Input: part model. Units: mm. Frame: model coordinates. Round coordinates to 2 decimals unless told otherwise and drop trailing zeros. Order: outer loops, then holes, each group sorted by start corner. A loop starts at its lowest first (then second) coordinate and runs counter-clockwise, first axis right, second up. Notation, with made-up numbers: (6.25, 47.25) -> (36.25, 47.25) arc R35 cw to (36.25, 84.25) -> close; hole circle Ø2 at (70.25, 43.5). An arc over 180 degrees is marked (long way). Use a Markdown table: item, result.
from build123d import *

# Parameters (mm, degrees)
ESQUISSE1_W                = 80
ESQUISSE1_H                = 30
BOSS_EXTRU_1_DEPTH         = 3
ESQUISSE2_W                = 10
ESQUISSE2_H                = 3
ENL_V_MAT_EXTRU_1_DEPTH    = 3
R_P_TITION_LIN_AIRE1_COUNT = 4
R_P_TITION_LIN_AIRE1_PITCH = 20
ESQUISSE3_W                = 3
ESQUISSE3_H                = 10
ENL_V_MAT_EXTRU_2_DEPTH    = 3


with BuildPart() as part:
    # Esquisse1 → Boss.-Extru.1 (new body)
    with BuildSketch(Plane.XY):
        with Locations((40, -15)):
            Rectangle(ESQUISSE1_W, ESQUISSE1_H)
    extrude(amount=BOSS_EXTRU_1_DEPTH)

    # Esquisse2 → Enlèv. mat.-Extru.1 (cut)
    with BuildSketch(Plane.XY.offset(3)):
        with Locations((75, -1.5)):
            Rectangle(ESQUISSE2_W, ESQUISSE2_H)
    enl_v_mat_extru_1 = extrude(amount=-ENL_V_MAT_EXTRU_1_DEPTH, mode=Mode.SUBTRACT)

    # Répétition linéaire1: Enlèv. mat.-Extru.1 ×4
    with Locations(*[(-i * R_P_TITION_LIN_AIRE1_PITCH, 0, 0) for i in range(1, R_P_TITION_LIN_AIRE1_COUNT)]):
        add(enl_v_mat_extru_1, mode=Mode.SUBTRACT)

    # Esquisse3 → Enlèv. mat.-Extru.2 (cut)
    with BuildSketch(Plane(origin=(0, 0, 0), x_dir=(-1, 0, 0), z_dir=(0, 0, -1))):
        with Locations((-1.5, -15)):
            Rectangle(ESQUISSE3_W, ESQUISSE3_H)
    extrude(amount=-ENL_V_MAT_EXTRU_2_DEPTH, mode=Mode.SUBTRACT)


solid = part.part
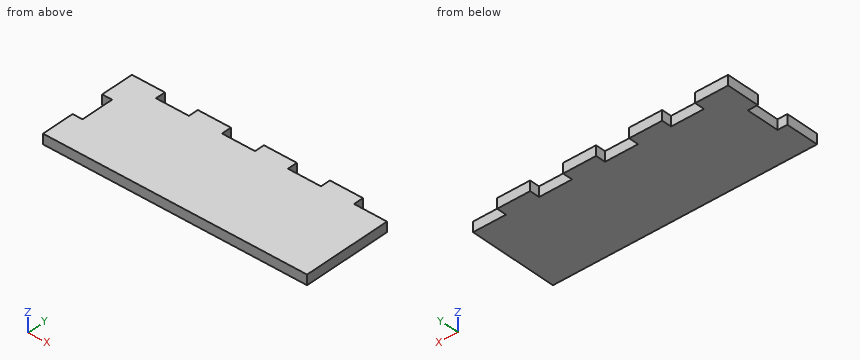
1) Contact query for flat-ended pins moving along their axis: P1, Ø1.5, axis at y = -2, z = 1.5, coming from the +X side; P2, Ø1.5, axis at y = -16.5, z = 2, coming from the -X side. Output: stop coordinate, or through.
Answer key:
| item | result |
|---|---|
| P1 | stops at x = 70 |
| P2 | stops at x = 3 |
2) Ray query, probe 1 along Y at (x, z) = (57.5, 0.4); probe 2 along X at (y, z) = (-15.25, 1.65). Return the intervals inside material, ascending.
Answer key:
| item | result |
|---|---|
| probe 1 | y = -30 to -3 |
| probe 2 | x = 3 to 80 |
3) Cut plane C-C on x = 59. Return loops of the section in (y, z), and give its area (3 significant figures).
Answer key:
| item | result |
|---|---|
| outline | (-30, 0) -> (-3, 0) -> (-3, 3) -> (-30, 3) -> close |
| area | 81.0 mm^2 |
4) Cut plane A-A on z = 0.8. Return loops of the section in (x, y), and give its area (3 significant figures).
Answer key:
| item | result |
|---|---|
| outline | (0, -30) -> (80, -30) -> (80, -3) -> (70, -3) -> (70, 0) -> (60, 0) -> (60, -3) -> (50, -3) -> (50, 0) -> (40, 0) -> (40, -3) -> (30, -3) -> (30, 0) -> (20, 0) -> (20, -3) -> (10, -3) -> (10, 0) -> (0, 0) -> (0, -10) -> (3, -10) -> (3, -20) -> (0, -20) -> close |
| area | 2,250 mm^2 |
5) Cut plane B-B on y = -17.75. Return loops of the section in (x, z), and give its area (3 significant figures).
Answer key:
| item | result |
|---|---|
| outline | (3, 0) -> (80, 0) -> (80, 3) -> (3, 3) -> close |
| area | 231 mm^2 |
